Verification items for the finished model (mm, model axes). A direction names the side the tool comes from. Coordinates: 2 decimals unless noted, no trailing zeros. Order: outer loops, then holes, each group sorted by start corner. A loop starts at its lowest first (then second) coordinate and runs counter-clockwise, first axis right, second up.
Q1. Cross-section at D-D, the plane x = 26.5. Record the boundary of the cut face in (y, z), and give its area (4 significant figures).
Q2. Draft check along X on faces 1 (the flat face through (25, -7, -4)), 2 (the cylindrical face through (-12, -3, 2)), 3 (the flat face through (-37.5, -3, 0)), 4 (the flat face through (37.5, -3, 0)). Enter one of: pulls with the +X half, pulls with the -X half, needs draft (parallel to the pull), parting line crosses it, or undercut.
Q3. Cross-section at C-C, the plane z = -14.5. Record the boundary of the cut face in (x, y).
Q4. Set-up check for faces 5 (the flat face through (25, -7, -17)), 6 (the flat face through (17.5, -7, -11)), 7 (the flat face through (32.5, -7, -11)), 8 (the flat face through (34, -6.5, 13)): record each of +Z, -Z, +X, -X, +Y, -Y from which the full face is reachable in a straight line by a thin tool's end or side.
Q5. Thickness scan on line 1 (Z direction, x = -9.5, y = -4.7); line 2 (Y direction, x = 22.5, z = 15); line 3 (Z direction, x = -8.5, y = -4.5). Record the ranges inside material, lowest first.
Q6. Cross-section at A-A, the plane z = 2. Record the boundary of the cut face in (x, y).
Q7. Cross-section at B-B, the plane x = -9.5. Record the boundary of the cut face in (y, z), and give its area (3 significant figures).
Q8. Depth check by flat-ended pin: P1, Ø2, axis at x = 4.5, z = 4, coming from the -Y side; P2, Ø1.2, axis at y = -8, z = -12, coming from the +X side; P3, Ø0.6, axis at x = 5.5, y = -6.5, coming from the -Z side. Enter the tip coordinate at first touch or a pass-through.
from build123d import *

# Parameters (mm, degrees)
F0_W     = 75
F0_H     = 40
F0_R     = 2.5
F1_DEPTH = 6
F2_W     = 10
F2_H     = 5
F2_W_2   = 5
F2_H_2   = 6
F2_W_3   = 2
F2_H_3   = 2
F3_DEPTH = 0.5
F4_W     = 15
F4_H     = 13
F5_DEPTH = 2.5


with BuildPart() as f1:
    # F0 (on Front) → F1 (new body)
    with BuildSketch(Plane.XZ):
        Rectangle(F0_W, F0_H)
        with Locations((-9.5, 2)):
            Circle(F0_R, mode=Mode.SUBTRACT)
    extrude(amount=F1_DEPTH)

    # F2 (on face) → F3 (join)
    with BuildSketch(Plane.XZ.offset(6)):
        with Locations((5.5, 16.5)):
            Rectangle(F2_W, F2_H)
        with Locations((34, 13)):
            Rectangle(F2_W_2, F2_H_2)
        with Locations((-18.5, 12)):
            Rectangle(F2_W_3, F2_H_3)
    extrude(amount=F3_DEPTH)

    # F4 (on face) → F5 (join)
    with BuildSketch(Plane.XZ.offset(6)):
        with Locations((25, -10.5)):
            Rectangle(F4_W, F4_H)
    extrude(amount=F5_DEPTH)


solid = f1.part
Check values:
1. outline: (-8.5, -17) - (-6, -17) - (-6, -20) - (0, -20) - (0, 20) - (-6, 20) - (-6, -4) - (-8.5, -4) - close
1. area: 272.5 mm2
2. face 1: needs draft
2. face 2: undercut
2. face 3: pulls with the -X half
2. face 4: pulls with the +X half
3. outline: (-37.5, -6) - (17.5, -6) - (17.5, -8.5) - (32.5, -8.5) - (32.5, -6) - (37.5, -6) - (37.5, 0) - (-37.5, 0) - close
4. face 5: -Z, +X, -X, -Y
4. face 6: +Z, -Z, -X, -Y
4. face 7: -Z, +X, -Y
4. face 8: +Z, +X, -X, -Y
5. line 1: z = -20 to -0.5, 4.5 to 20
5. line 2: y = -6 to 0
5. line 3: z = -20 to -0.29, 4.29 to 20
6. outline: (-37.5, -6) - (-12, -6) - (-12, 0) - (-37.5, 0) - close; (-7, -6) - (37.5, -6) - (37.5, 0) - (-7, 0) - close
7. outline: (-6, -20) - (0, -20) - (0, -0.5) - (-6, -0.5) - close; (-6, 4.5) - (0, 4.5) - (0, 20) - (-6, 20) - close
7. area: 210 mm2
8. P1: stops at y = -6
8. P2: stops at x = 32.5
8. P3: stops at z = 14
